Verification items for the finished model (mm, model axes). Coordinates: 2 decimals unless noted, no trailing zeros. Write each loop counter-clockwise with the first axis right and the second up, starting at its lowest first coordinate (ties: lowest second). Pieces come first, ordered by that corner, then holes. Notation, with made-up numbers: M -30,82 L -8,82 A20 ccw -8,110 Z; hole C 7,-5.75 d8. An arc over 180 degrees is marked long. Answer in a Markdown table with one row per item.
from build123d import *

# Parameters (mm, degrees)
PAD015_DEPTH                        = 3
SKETCH054_R                         = 1.65
POCKET018_DEPTH                     = 358.938883
POCKET018_DEPTH_BACK                = 361.938883
BODY001003005003004_PLACEMENT_ANGLE = 60
CLONE007_PLACEMENT_ANGLE            = 25


with BuildPart() as part:
    # Sketch053 → Pad015 (new body)
    with BuildSketch(Plane.XY):
        with BuildLine():
            ThreePointArc((152.005097, 113.785532), (84.992984, 169.790723), (0, 189.875477))
            Line((0, 189.875477), (0, 196.875477))
            ThreePointArc((157.608957, 117.98038), (88.126358, 176.050273), (0, 196.875477))
            ThreePointArc((152.005097, 113.785532), (156.904451, 113.081026), (157.608957, 117.98038))
        make_face()
    pad015 = extrude(amount=PAD015_DEPTH)

    # Sketch054 → Pocket018 (cut, two sides)
    with BuildSketch(Plane.XY) as pocket018_sk:
        with Locations((150.82443, 121.020933)):
            Circle(SKETCH054_R)
        with BuildLine():
            ThreePointArc((0, 191.725477), (1.65, 193.375477), (0, 195.025477))
            Line((0, 191.725477), (0, 195.025477))
        make_face()
    pocket018 = extrude(amount=-POCKET018_DEPTH, mode=Mode.SUBTRACT) + extrude(pocket018_sk.sketch, amount=POCKET018_DEPTH_BACK, mode=Mode.SUBTRACT)

    # Mirrored020: Pad015, Pocket018 across Sketch053 V_Axis
    add(pad015.mirror(Plane(origin=(0, 0, 0), x_dir=(0, 0, 1), z_dir=(1, 0, 0))))
    add(pocket018.mirror(Plane(origin=(0, 0, 0), x_dir=(0, 0, 1), z_dir=(1, 0, 0))), mode=Mode.SUBTRACT)


with BuildPart() as part_1:
    # Body001003005003004 placement: moved
    add(part.part.rotate(Axis((0, 0, 0), (0, 0, 1)), BODY001003005003004_PLACEMENT_ANGLE))


with BuildPart() as part_2:
    # Clone007 placement: moved
    add(part_1.part.moved(Location((1071, 433, 0))).rotate(Axis((1071, 433, 0), (0, 0, -1)), CLONE007_PLACEMENT_ANGLE))


solid = part_2.part
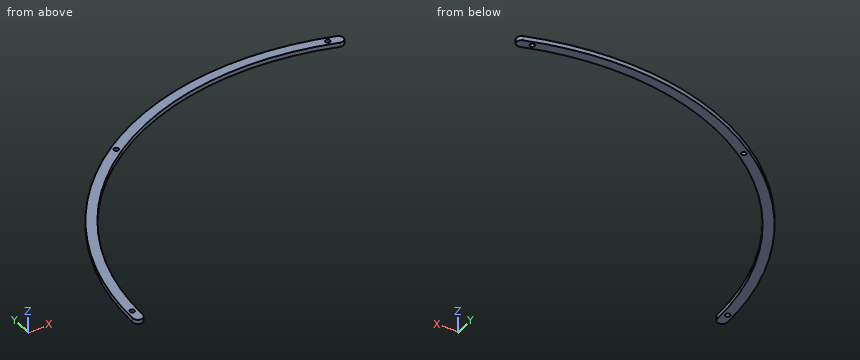
1) Thickness scan on L1, parallel to Y at x = 1070, z = 0.65; L2, parallel to Y at x = 946, z = 2.3; L3, parallel to X at y = 536, z = 1.4. Record the ranges inside material, lowest first. Write a range as [from, to].
Response values:
| item | result |
|---|---|
| L1 | y = [622.87, 629.87] |
| L2 | y = [575.93, 585.1] |
| L3 | x = [903.22, 911.49] |
2) Sectioned sample at A-A (z = 1.4). Record the cut outline in (x, y), then the cut area to 3 significant figures.
Response values:
| item | result |
|---|---|
| outline | M 874.22,439.24 A3.5 ccw 881.22,439.02 A189.88 cw 962.09,588.54 A189.88 cw 1130.25,613.39 A3.5 ccw 1132.43,620.04 A196.88 ccw 958.08,594.27 A196.88 ccw Z; hole C 878.04,445.63 d3.3; hole C 960.08,591.4 d3.3; hole C 1125.13,618.64 d3.3 |
| area | 2,530 mm² |
3) Depth check by flat-ended pin: pin 1 (1 mm diameter, centred on x = 1020, z = 2, fed in from -Y). Enter the tip coordinate at first touch or a pass-through.
Response values:
| item | result |
|---|---|
| pin 1 | stops at y = 615.76 |
4) Sectioned sample at C-C (x = 1031). Record the cut outline in (y, z).
Response values:
| item | result |
|---|---|
| outline | M 618.61,0 L 625.77,0 L 625.77,3 L 618.61,3 Z |
5) Sectioned sample at B-B (y = 465). Record the cut outline in (x, z), then the cut area to 3 significant figures.
Response values:
| item | result |
|---|---|
| outline | M 876.74,0 L 883.84,0 L 883.84,3 L 876.74,3 Z |
| area | 21.3 mm² |
